```python
from build123d import *

# Parameters (mm, degrees)
F0_W      = 38.1
F0_H      = 38.1
F6_DEPTH  = 38.1
F7_DEPTH  = 38.1
F8_DEPTH  = 38.1
F9_W      = 25.4
F9_H      = 7.62
F10_DEPTH = 38.1


with BuildPart() as f6:
    # F0 (on Front) → F6 (new body)
    with BuildSketch(Plane.XZ):
        with Locations((19.05, 19.05)):
            Rectangle(F0_W, F0_H)
    extrude(amount=F6_DEPTH)

    # F4 (on offset) → F7 (cut)
    with BuildSketch(Plane.YZ.offset(38.1)):
        Polygon((-31.75, 0), (-38.1, 38.1), (-38.1, 0), align=None)
        Polygon((-6.35, 38.1), (-31.75, 38.1), (-26.67, 15.875), (-21.59, 28.575), (-16.51, 28.575), (-11.43, 15.875), align=None)
        Polygon((-19.05, 15.875), (-25.4, 0), (-12.7, 0), align=None)
        Polygon((0, 0), (0, 38.1), (-6.35, 0), align=None)
    extrude(amount=-F7_DEPTH, mode=Mode.SUBTRACT)

    # F5 (on offset) → F8 (cut)
    with BuildSketch(Plane.XZ.offset(38.1)):
        Polygon((0, 38.1), (0, 0), (6.35, 38.1), align=None)
        Polygon((25.4, 38.1), (12.7, 38.1), (19.05, 22.225), align=None)
        Polygon((31.75, 38.1), (38.1, 0), (38.1, 38.1), align=None)
        Polygon((11.43, 22.225), (6.35, 0), (31.75, 0), (26.67, 22.225), (21.59, 9.525), (16.51, 9.525), align=None)
    extrude(amount=-F8_DEPTH, mode=Mode.SUBTRACT)

    # F9 (on offset) → F10 (cut)
    with BuildSketch(Plane.XY.offset(38.1)):
        with Locations((25.4, -11.43)):
            Rectangle(F9_W, F9_H)
        with Locations((12.7, -26.67)):
            Rectangle(F9_W, F9_H)
    extrude(amount=-F10_DEPTH, mode=Mode.SUBTRACT)


solid = f6.part
```
Geometry check sheet. Reference: the model listing, model coordinates, mm. A direction names the side the tool comes from. Give positions to 0.01 mm unless a question says otherwise; leave off trailing zeros. Write each loop counter-clockwise with the first axis right and the second up, starting at its lowest first coordinate (ties: lowest second). Pieces come first, ordered by that corner, then holes.
1) Access from +Z, -Z, +X, -X, +Y, -Y to the whole of each face (thin tool, end or side, straight path). Record for faces 1 (the flat face through (5.06, -15.83, 7.83)), 2 (the flat face through (19, -22, 9.525)), 3 (the flat face through (12.7, -8, 23)), 4 (the flat face through (25.4, -30, 23)).
2) Release check for a two-part mould opening along X. For faces 5 (the flat face through (3.836, -33.497, 23.017)), 6 (the flat face through (19, -6, 9.525)), 7 (the flat face through (11, -19, 28.575)) record: pulls with the +X half, pulls with the -X half, needs draft (parallel to the pull), parting line crosses it, or undercut.
3) Section check B-B, the plane x = 15.5. Record the boundary of the cut face in (y, z) (3 decimals), and give its area (3 significant figures).
4) Section check D-D, the plane z = 26. Record the boundary of the cut face in (x, y), and give its area (3 significant figures).
5) Section check A-A, the plane z = 36. Record the boundary of the cut face in (x, y).
6) Gauge pin test, flat ends, axial feed: pin 1 (5.5 mm diameter, centred on x = 10, z = 18, fed in from -Y); pin 2 (6 mm diameter, centred on y = -18, z = 24, fed in from -X); pin 3 (12.5 mm diameter, centred on x = 8, z = 17.5, fed in from +Y); pin 4 (12 mm diameter, centred on x = 20, y = -33.5, fed in from +Z). Record the tip position at first contact, or that the pin passes through.
7) Material ranges on L1, parallel to Y at x = 17, z = 27; L2, parallel to Y at x = 32, z = 28.5; L3, parallel to Y at x = 19, z = 12.5, recorded low to high.
Computed:
1. face 1: -Z, +X, -X
1. face 2: -Z, +Y, -Y
1. face 3: +Z, -Z, +X
1. face 4: +Z, -Z, -X
2. face 5: pulls with the -X half
2. face 6: undercut
2. face 7: needs draft
3. outline: (-36.933, 31.1) - (-33.758, 12.05) - (-30.48, 12.05) - (-30.48, 31.1) - close; (-22.86, 12.05) - (-20.58, 12.05) - (-19.05, 15.875) - (-17.52, 12.05) - (-15.24, 12.05) - (-15.24, 25.4) - (-16.51, 28.575) - (-21.59, 28.575) - (-22.86, 25.4) - close; (-7.62, 12.05) - (-4.342, 12.05) - (-1.167, 31.1) - (-7.62, 31.1) - close
3. area: 301 mm2
4. outline: (4.33, -36.08) - (17.54, -36.08) - (17.54, -30.48) - (4.33, -30.48) - close; (4.33, -22.62) - (17.54, -22.62) - (17.54, -15.48) - (4.33, -15.48) - close; (4.33, -9.12) - (12.7, -9.12) - (12.7, -7.62) - (17.54, -7.62) - (17.54, -2.02) - (4.33, -2.02) - close; (20.56, -36.08) - (33.77, -36.08) - (33.77, -28.98) - (25.4, -28.98) - (25.4, -30.48) - (20.56, -30.48) - close; (20.56, -22.62) - (33.77, -22.62) - (33.77, -15.48) - (20.56, -15.48) - close; (20.56, -7.62) - (33.77, -7.62) - (33.77, -2.02) - (20.56, -2.02) - close
4. area: 510 mm2
5. outline: (6, -37.75) - (13.54, -37.75) - (13.54, -31.27) - (6, -31.27) - close; (6, -6.83) - (13.54, -6.83) - (13.54, -0.35) - (6, -0.35) - close; (24.56, -37.75) - (32.1, -37.75) - (32.1, -31.27) - (24.56, -31.27) - close; (24.56, -6.83) - (32.1, -6.83) - (32.1, -0.35) - (24.56, -0.35) - close
6. pin 1: stops at y = -35.21
6. pin 2: stops at x = 3.5
6. pin 3: stops at y = -2.39
6. pin 4: stops at z = 38.1
7. L1: y = -36.25 to -30.48, -22.22 to -15.88, -7.62 to -1.85
7. L2: y = -36.5 to -29.56, -21.62 to -16.48, -7.62 to -1.6
7. L3: y = -33.83 to -30.48, -22.86 to -20.4, -17.7 to -15.24, -7.62 to -4.27
